```python
from build123d import *

# Parameters (mm, degrees)
F0_R     = 16.75
F1_DEPTH = 10


with BuildPart() as f1:
    # F0 (on Top) → F1 (new body)
    with BuildSketch(Plane.XY):
        with BuildLine():
            ThreePointArc((-20.206893, -4.716353), (20.75, 0), (-20.206893, 4.716353))
            ThreePointArc((-20.206893, 4.716353), (-29.246043, 0), (-20.206893, -4.716353))
        make_face()
        with BuildLine():
            ThreePointArc((-20.749537, -0.138584), (-26.246043, 0), (-20.749537, 0.138584))
            ThreePointArc((-20.749537, 0.138584), (-20.746917, 0.069314), (-20.746043, 0))
            ThreePointArc((-20.746043, 0), (-20.746917, -0.069314), (-20.749537, -0.138584))
        make_face(mode=Mode.SUBTRACT)
        Circle(F0_R, mode=Mode.SUBTRACT)
    extrude(amount=F1_DEPTH)


solid = f1.part
```
The listing builds one solid part. Answer for the finished solid, in the listing's coordinates (mm). Coordinates: 2 decimals unless noted, no trailing zeros. Write each loop counter-clockwise with the first axis right and the second up, starting at its lowest first coordinate (ties: lowest second). Pieces come first, ordered by that corner, then holes. Notation, with made-up numbers: M 21.25,-25.5 L 30.25,-25.5 A22 cw 30.25,0.5 Z; hole C 64,48 d5. An arc over 180 degrees is marked long. Use a Markdown table: item, result. Add a question column.
1. Section B-B (y = 1) is taken. Give the vertices of the cut face in (x, z).
2. For a pull along Y with two mould halves and no side action, classify faces 1 (the cylindrical face through (-3.63, -16.35, 4.93)), 2 (the flat face through (-17, 0, 10)), 3 (the cylindrical face through (-26.243, -0.119, 4.93)), 4 (the cylindrical face through (20.733, -0.846, 4.93)) as +Y half, -Y half, draft (parallel to the pull), parting line (faces both ways), or undercut.
3. Section A-A (x = -8.5) is taken. Give the vertices of the cut face in (y, z), plus the area to 3 significant figures.
4. Section C-C (z = 4.25) is taken. Give the vertices of the cut face in (x, y), plus the area to 3 significant figures.
5. Given P1, Ø3, axis at x = -14.5, z = 3.5, coming from the +Y side; P2, Ø1.5, axis at x = -7, z = 8, coming from the +Y side; P3, Ø20, axis at x = 0, y = 0, coming from the +Z side; P4, Ø10, axis at x = -13, y = 0.5, coming from the -Z side, each flat-ended and moving along its own axis, determine where each tip first touches the part or whether it passes through.
6. Straight lines are drawn through the part: line 1 along Y through (x, z) = (0, 7.5); line 2 along Y through (x, z) = (6.5, 7.5); line 3 along X through (y, z) = (12, 8.5). For each, find the intervals that lie inside material, in ascending order. Write a range as [from, to].
7. Section D-D (x = 0) is taken. Give the vertices of the cut face in (y, z).
Data:
| question | item | result |
|---|---|---|
| 1 | outline | M -29.16,0 L -26.06,0 L -26.06,10 L -29.16,10 Z; M -20.93,0 L -16.72,0 L -16.72,10 L -20.93,10 Z; M 16.72,0 L 20.73,0 L 20.73,10 L 16.72,10 Z |
| 2 | face 1 | undercut |
| 2 | face 2 | draft |
| 2 | face 3 | undercut |
| 2 | face 4 | parting line |
| 3 | outline | M -18.93,0 L -14.43,0 L -14.43,10 L -18.93,10 Z; M 14.43,0 L 18.93,0 L 18.93,10 L 14.43,10 Z |
| 3 | area | 89.9 mm2 |
| 4 | outline | M -20.21,-4.72 A20.75 ccw long -20.21,4.72 A5.75 ccw long Z; hole M -20.75,-0.14 A2.75 ccw -20.75,0 A2.75 ccw -20.75,0.14 A2.75 ccw long Z; hole C 0,0 d33.5 |
| 4 | area | 532 mm2 |
| 5 | P1 | stops at y = 16.17 |
| 5 | P2 | stops at y = 19.79 |
| 5 | P3 | passes through |
| 5 | P4 | stops at z = 0 |
| 6 | line 1 | y = [-20.75, -16.75], [16.75, 20.75] |
| 6 | line 2 | y = [-19.71, -15.44], [15.44, 19.71] |
| 6 | line 3 | x = [-16.93, -11.69], [11.69, 16.93] |
| 7 | outline | M -20.75,0 L -16.75,0 L -16.75,10 L -20.75,10 Z; M 16.75,0 L 20.75,0 L 20.75,10 L 16.75,10 Z |
